Source: three-view drawing plus pictorial views. Frame: mm from the lowest corner of the part. A direction names the side the tool comes from. Coordinates: 2 decimals unless noted, no trailing zeros. Write each loop counter-clockwise with the first axis right and the second up, starting at its lowest first coordinate (ties: lowest second). Pieces come first, ordered by that corner, then holes. Notation, with made-up numbers: (80.5, 11.5) -> (107.5, 11.5) arc R20 cw to (107.5, 35.5) -> close; hole circle Ø4 at (30, -8.75). An arc over 180 degrees is marked (long way). Write item = value, one per line.
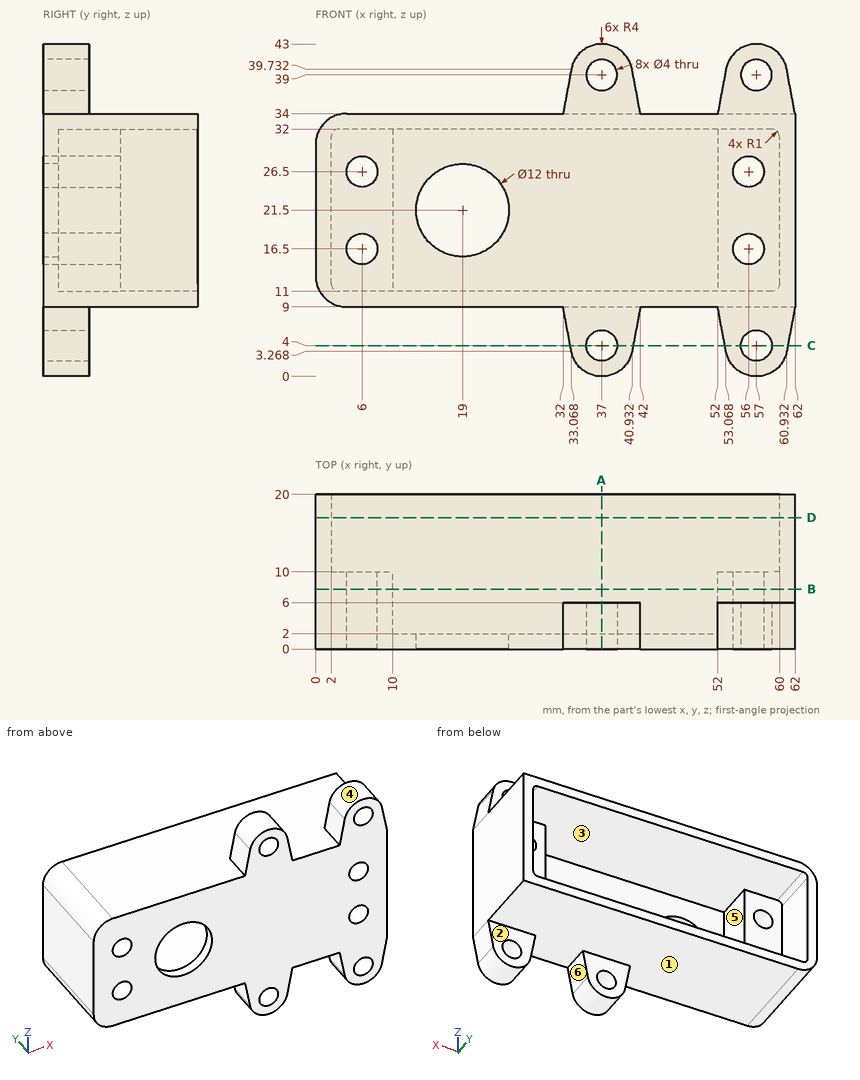
1) First-contact query: pin 1 Ø7 at (x, z) = (56, 40.5) entering from +Y; pin 2 Ø12 at (x, y) = (53, 17) entering from -Z; pin 3 Ø6.5 at (x, z) = (6, 16.5) entering from +Y. Flat tips, straight axial feed; report the tip coordinate or a pass-through.
Answer block:
pin_1 = 6
pin_2 = 9
pin_3 = 10
2) Cut plane D-D, the plane y = 17. Output: boundary loops of the cut face in (x, z), and give its area (3 significant figures).
Answer block:
outline = (0, 13) arc R4 ccw to (4, 9) -> (62, 9) -> (62, 34) -> (4, 34) arc R4 ccw to (0, 30) -> close; hole (2, 12) arc R1 ccw to (3, 11) -> (59, 11) arc R1 ccw to (60, 12) -> (60, 31) arc R1 ccw to (59, 32) -> (3, 32) arc R1 ccw to (2, 31) -> close
area = 326 mm2
3) Cut plane A-A, the plane x = 37. Output: boundary loops of the cut face in (y, z).
Answer block:
outline = (0, 0) -> (6, 0) -> (6, 2) -> (0, 2) -> close; (0, 6) -> (6, 6) -> (6, 9) -> (20, 9) -> (20, 11) -> (2, 11) -> (2, 32) -> (20, 32) -> (20, 34) -> (6, 34) -> (6, 37) -> (0, 37) -> close; (0, 41) -> (6, 41) -> (6, 43) -> (0, 43) -> close
4) Cut plane C-C, the plane z = 4. Output: boundary loops of the cut face in (x, y).
Answer block:
outline = (32.93, 0) -> (35, 0) -> (35, 6) -> (32.93, 6) -> close; (39, 0) -> (41.07, 0) -> (41.07, 6) -> (39, 6) -> close; (52.93, 0) -> (55, 0) -> (55, 6) -> (52.93, 6) -> close; (59, 0) -> (61.07, 0) -> (61.07, 6) -> (59, 6) -> close
5) Cut plane B-B, the plane y = 7.75. Output: boundary loops of the cut face in (x, z).
Answer block:
outline = (0, 13) arc R4 ccw to (4, 9) -> (62, 9) -> (62, 34) -> (4, 34) arc R4 ccw to (0, 30) -> close; hole circle Ø4 at (6, 16.5); hole circle Ø4 at (6, 26.5); hole (10, 11) -> (52, 11) -> (52, 32) -> (10, 32) -> close; hole circle Ø4 at (56, 16.5); hole circle Ø4 at (56, 26.5)
6) Pull-direction query (Z, two-part tool) for the marked faces 1, 2 and 3; classes: +Z half, -Z half, draft (parallel to the pull), parting line (faces both ways), or undercut.
Answer block:
face_1 = -Z half
face_2 = draft
face_3 = undercut
7) Material intervals for probe 1 along X at (y, z) = (2.25, 22.5); probe 2 along Z at (x, y) = (19, 12); probe 3 along X at (y, z) = (8.75, 26), sorted ascending. Write a range as [from, to].
Answer block:
probe_1 = [0, 10], [52, 62]
probe_2 = [9, 11], [32, 34]
probe_3 = [0, 4.06], [7.94, 10], [52, 54.06], [57.94, 62]
8) Reachability of the marked faces 4, 5 and 6 from +Z, -Z, +X, -X, +Y, -Y: full face, straight path, thin tool, end or side. Return the list, or none.
Answer block:
face_4 = +Z, +Y, -Y
face_5 = +Y
face_6 = -Z, +Y, -Y
